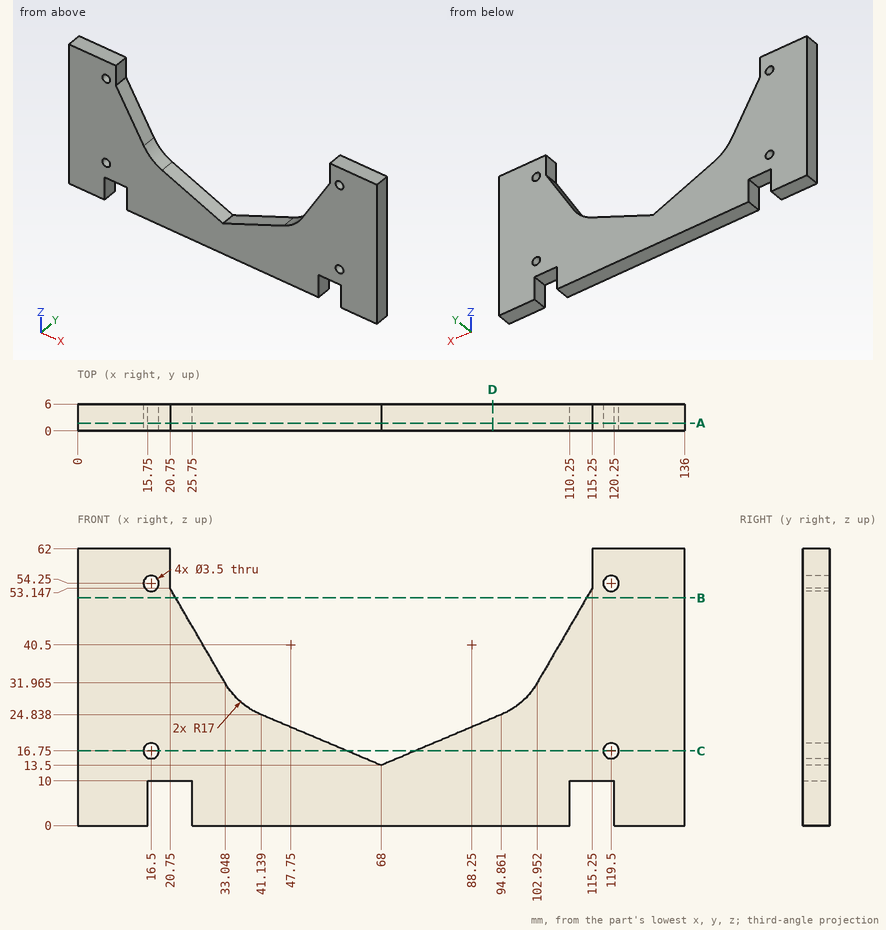
The drawing under review shows one solid part. Ordinate dimensions are in mm from its lowest x, y, z. Coordinates: 2 decimals unless noted, no trailing zeros. Order: outer loops, then holes, each group sorted by start corner. A loop starts at its lowest first (then second) coordinate and runs counter-clockwise, first axis right, second up. Notation, with made-up numbers: (71, 33) -> (79, 33) arc R16 ccw to (79, 54) -> close; hole circle Ø7 at (79, 77.25). An arc over 180 degrees is marked (long way). Answer in a Markdown table with one row per item.
(1) Consider section C-C (z = 16.75). Write out the cut boundary in (x, y).
Answers:
| item | result |
|---|---|
| outline | (0, 0) -> (14.75, 0) -> (14.75, 6) -> (0, 6) -> close; (18.25, 0) -> (60.3, 0) -> (60.3, 6) -> (18.25, 6) -> close; (75.7, 0) -> (117.75, 0) -> (117.75, 6) -> (75.7, 6) -> close; (121.25, 0) -> (136, 0) -> (136, 6) -> (121.25, 6) -> close |
(2) Consider section A-A (y = 1.7). State how many separate pieces and enclosed holes the cut face has, plus the area to 3 significant figures.
Answers:
| item | result |
|---|---|
| separate pieces | 1 |
| enclosed holes | 4 |
| area | 4,860 mm² |
(3) Consider section B-B (z = 51). Write out the cut boundary in (x, y), plus the area to 3 significant figures.
Answers:
| item | result |
|---|---|
| outline | (0, 0) -> (22, 0) -> (22, 6) -> (0, 6) -> close; (114, 0) -> (136, 0) -> (136, 6) -> (114, 6) -> close |
| area | 264 mm² |
(4) Wall thickness on line 1 along Z through (x, y) = (16.5, 3); line 2 along X through (y, z) = (4.1, 8); line 3 along X through (y, z) = (5.7, 17) (1 decimal): over which ranges is each line inside the solid? List them lowest first.
Answers:
| item | result |
|---|---|
| line 1 | 10 to 15, 18.5 to 52.5, 56 to 62 |
| line 2 | 0 to 15.75, 25.75 to 110.25, 120.25 to 136 |
| line 3 | 0 to 14.8, 18.2 to 59.7, 76.3 to 117.8, 121.2 to 136 |
(5) Insertion check: pin 1 (1.8 mm diameter, centred on x = 20.5, y = 1.5, fed in from -Z). The pin has a flat end and moves straight along its axis. Give the tip position at first contact, or say it passes through.
Answers:
| item | result |
|---|---|
| pin 1 | z = 10 |
(6) Consider section D-D (x = 93). Write out the cut boundary in (y, z), plus the area to 3 significant figures.
Answers:
| item | result |
|---|---|
| outline | (0, 0) -> (6, 0) -> (6, 24.05) -> (0, 24.05) -> close |
| area | 144 mm² |
